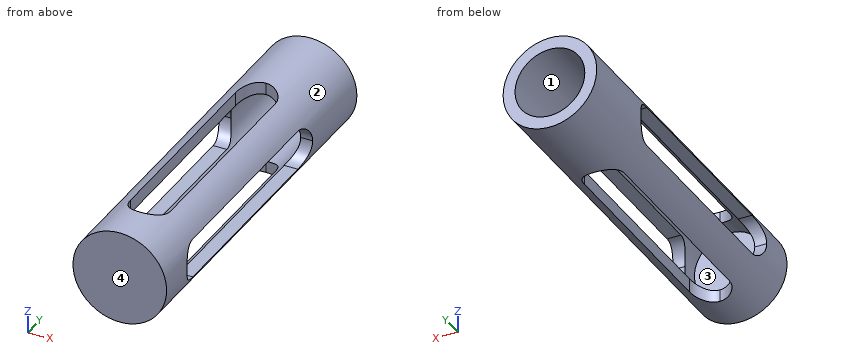
```python
from build123d import *

# Parameters (mm, degrees)
F0_R     = 4.7
F1_DEPTH = 36.6
F2_R     = 3.5
F3_DEPTH = 34.5
F4_W     = 4
F4_H     = 24.2
F5_DEPTH = 12.5
F6_W     = 24.2
F6_H     = 4
F7_DEPTH = 12.5
F8_R     = 1.9999


# Not quite as in the source:
# - a fillet or chamfer is up to 0.001 mm smaller than in the source, because OpenCascade refuses the exact size


with BuildPart() as f1:
    # F0 (on Front) → F1 (new body)
    with BuildSketch(Plane.XZ):
        Circle(F0_R)
    extrude(amount=F1_DEPTH)

    # F2 (on face) → F3 (cut)
    with BuildSketch(Plane(origin=(0, 0, 0), x_dir=(-1, 0, 0), z_dir=(0, 1, 0))):
        Circle(F2_R)
    extrude(amount=-F3_DEPTH, mode=Mode.SUBTRACT)

    # F4 (on Top) → F5 (cut, symmetric)
    with BuildSketch(Plane.XY):
        with Locations((0, -20.6)):
            Rectangle(F4_W, F4_H)
    extrude(amount=F5_DEPTH, both=True, mode=Mode.SUBTRACT)

    # F6 (on Right) → F7 (cut, symmetric)
    with BuildSketch(Plane.YZ):
        with Locations((-20.6, 0)):
            Rectangle(F6_W, F6_H)
    extrude(amount=F7_DEPTH, both=True, mode=Mode.SUBTRACT)

    # F8 (radius 2 in the source; OpenCascade refuses exactly that, so slightly less here)
    f8_edges = [f1.edges().sort_by_distance(p)[0] for p in [
        (2, -8.5, 3.562758),
        (2, -8.5, -3.562758),
        (-2, -8.5, 3.562758),
        (-2, -8.5, -3.562758),
        (3.562758, -8.5, -2),
        (-3.562758, -8.5, -2),
        (3.562758, -8.5, 2),
        (-3.562758, -8.5, 2),
        (3.562758, -32.7, 2),
        (-3.562758, -32.7, 2),
        (3.562758, -32.7, -2),
        (-3.562758, -32.7, -2),
        (-2, -32.7, 3.562758),
        (-2, -32.7, -3.562758),
        (2, -32.7, 3.562758),
        (2, -32.7, -3.562758),
    ]]
    fillet(f8_edges, radius=F8_R)


solid = f1.part
```
Read the model definition and answer for the solid it produces. Units are mm, in the model's axes. Face numbers are marked on the shaded views. Coordinates: 2 decimals unless noted, no trailing zeros. Write each loop counter-clockwise with the first axis right and the second up, starting at its lowest first coordinate (ties: lowest second). Pieces come first, ordered by that corner, then holes. Notation, with made-up numbers: (-6.75, 19.25) -> (23.25, 19.25) arc R14 cw to (23.25, 34.25) -> close; hole circle Ø8 at (-28, -36.75). An arc over 180 degrees is marked (long way). Return JSON: item names as keys, results as strings.
1. A cutting plane is placed at C-C (y = -7). Determine the outline of the cut face in (x, z), and give its area (3 significant figures).
Found:
{"outline": "circle Ø9.4 at (0, 0); hole circle Ø7 at (0, 0)", "area": "30.9 mm2"}
2. Find the intervals of material crossed by line 1 along X through (y, z) = (-8, 0); line 2 along X through (y, z) = (-2.5, -2.25); line 3 along Y through (x, z) = (-1, 1.5), in increasing order. Write a range as from..to.
Found:
{"line 1": "-4.7..-3.5, 3.5..4.7", "line 2": "-4.13..-2.68, 2.68..4.13", "line 3": "-36.6..-34.5"}
3. Determine the mould class of the marked faces 1, 2, 3 and 4 for opening direction X: pulls with the +X half, pulls with the -X half, needs draft (parallel to the pull), parting line crosses it, or undercut.
Found:
{"face 1": "undercut", "face 2": "parting line crosses it", "face 3": "undercut", "face 4": "needs draft"}
4. A cutting plane is placed at A-A (y = -27). Determine the outline of the cut face in (x, z), and give its area (3 significant figures).
Found:
{"outline": "(-4.25, -2) arc R4.7 ccw to (-2, -4.25) -> (-2, -2.87) arc R3.5 cw to (-2.87, -2) -> close; (-4.25, 2) -> (-2.87, 2) arc R3.5 cw to (-2, 2.87) -> (-2, 4.25) arc R4.7 ccw to start; (2, -4.25) arc R4.7 ccw to (4.25, -2) -> (2.87, -2) arc R3.5 cw to (2, -2.87) -> close; (2, 2.87) arc R3.5 cw to (2.87, 2) -> (4.25, 2) arc R4.7 ccw to (2, 4.25) -> close", "area": "10.8 mm2"}
5. A cutting plane is placed at B-B (z = 0.5). Determine the outline of the cut face in (x, y), and give its area (3 significant figures).
Found:
{"outline": "(-4.67, -36.6) -> (4.67, -36.6) -> (4.67, -32.64) -> (3.46, -32.64) -> (3.46, -34.5) -> (-3.46, -34.5) -> (-3.46, -32.64) -> (-4.67, -32.64) -> close; (-4.67, -8.56) -> (-3.46, -8.56) -> (-3.46, 0) -> (-4.67, 0) -> close; (3.46, -8.56) -> (4.67, -8.56) -> (4.67, 0) -> (3.46, 0) -> close", "area": "44.8 mm2"}
6. Each of these flat-tipped pins is pushed along its axis until it touches: P1, Ø3, axis at x = -1, y = -22.5, coming from the +Z side; P2, Ø0.7, axis at y = -17.5, z = 4, coming from the +X side; P3, Ø1.1, axis at y = -19, z = -3.5, coming from the -X side. Where does it stop, or does it pass through?
Found:
{"P1": "z = 4.25", "P2": "x = 2.96", "P3": "x = -3.66"}
